Autodesk Inventor part; units mm, degrees
ref_plane "YZ Plane" through (0, 0, 0) normal (1, 0, 0) x (0, 1, 0)
ref_plane "XZ Plane" through (0, 0, 0) normal (0, 1, 0) x (-1, 0, 0)
ref_plane "XY Plane" through (0, 0, 0) normal (0, 0, 1) x (1, 0, 0)
sketch "Sketch2" plane through (0, 0, 0) normal (0, 0, 1) x (1, 0, 0)
  circle A0 centre (0, 0) radius 3.75
  circle A1 centre (0, 0) radius 2
  dimension "d6" = 7.5
  dimension "d7" = 4
extrude "Extrusion1" add sketch "Sketch2" along normal blind 6
sketch "Sketch3" plane through (0, 0, 0) normal (0, 0, -1) x (-1, 0, 0)
  line L0 (-12, -4) -> (12, -4)
  line L1 (12, -4) -> (12, 12)
  line L2 (12, 12) -> (-12, 12)
  line L3 (-12, 12) -> (-12, -4)
  line L4 (0, 0) -> (0, 4.4651)
  line L5 (0, 4.4651) -> (0, 0)
  line L6 (0, 0) -> (5, 0)
  circle A0 centre (0, 0) radius 2
  circle A1 centre (0, 0) radius 2
  dimension "d10" = 24
  dimension "d11" = 16
  dimension "d12" = 4
extrude "Extrusion4" add sketch "Sketch3" against normal blind 2
properties part number "fijador.rodamiento"
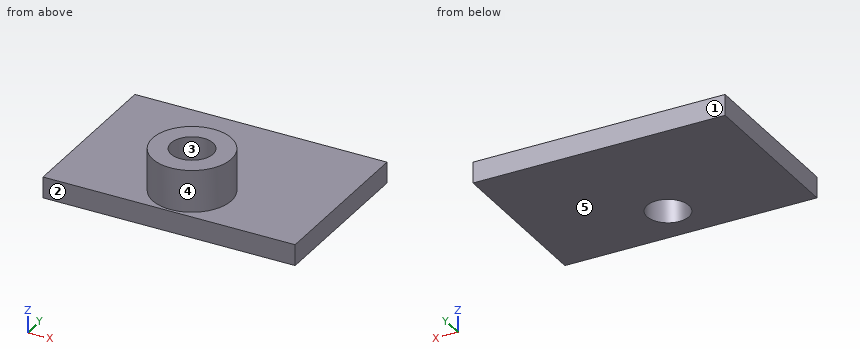
Geometry check sheet. Reference: the model listing, model coordinates, mm. Face numbers are marked on the shaded views. A direction names the side the tool comes from. Give positions to 0.01 mm unless a question says otherwise; leave off trailing zeros. Order: outer loops, then holes, each group sorted by start corner. A loop starts at its lowest first (then second) coordinate and runs counter-clockwise, first axis right, second up. Notation, with made-up numbers: (18.5, -22.75) - (44.5, -22.75) arc R9 cw to (44.5, -11.75) - close; hole circle Ø9 at (51.25, 41). An arc over 180 degrees is marked (long way). Use one line per item in the form item = value.
1) Material ranges on probe 1 along Y at (x, z) = (0, 3.3); probe 2 along Y at (x, z) = (0, 1.4); probe 3 along Z at (x, y) = (-7.75, 11), recorded low to high. Write a range as from..to.
Working result:
probe_1 = -3.75..-2, 2..3.75
probe_2 = -4..-2, 2..12
probe_3 = 0..2
2) Sectioned sample at D-D (y = -2.5). Record the boundary of the cut face in (x, z).
Working result:
outline = (-12, 0) - (12, 0) - (12, 2) - (2.8, 2) - (2.8, 6) - (-2.8, 6) - (-2.8, 2) - (-12, 2) - close
3) Depth check by flat-ended pin: pin 1 Ø3 at (x, y) = (-7, 4.5) entering from +Z. Enter the tip coordinate at first touch or a pass-through.
Working result:
pin_1 = 2
4) Access from +Z, -Z, +X, -X, +Y, -Y to the whole of each face (thin tool, end or side, straight path). Record for the marked faces 4 and 5.
Working result:
face_4 = +Z
face_5 = -Z, +X, -X, +Y, -Y
5) Sectioned sample at C-C (z = 5.3). Record the boundary of the cut face in (x, y).
Working result:
outline = circle Ø7.5 at (0, 0); hole circle Ø4 at (0, 0)
6) Sectioned sample at B-B (y = 0). Record the boundary of the cut face in (x, z).
Working result:
outline = (-12, 0) - (-2, 0) - (-2, 6) - (-3.75, 6) - (-3.75, 2) - (-12, 2) - close; (2, 0) - (12, 0) - (12, 2) - (3.75, 2) - (3.75, 6) - (2, 6) - close
7) Draft check along Y on the marked faces 1, 2 and 3. Enter one of: released by +Y, released by -Y, zero draft, split by the parting line, or undercut.
Working result:
face_1 = released by +Y
face_2 = released by -Y
face_3 = undercut
8) Sectioned sample at A-A (x = 0). Record the boundary of the cut face in (y, z).
Working result:
outline = (-4, 0) - (-2, 0) - (-2, 6) - (-3.75, 6) - (-3.75, 2) - (-4, 2) - close; (2, 0) - (12, 0) - (12, 2) - (3.75, 2) - (3.75, 6) - (2, 6) - close
